For this review, use the dimensioned drawing (mm, ordinates from the lowest corner) and the shaded views. A direction names the side the tool comes from. Coordinates: 2 decimals unless noted, no trailing zeros. Order: outer loops, then holes, each group sorted by start corner. A loop starts at its lowest first (then second) coordinate and runs counter-clockwise, first axis right, second up. Notation, with made-up numbers: M 78.5,15.5 L 118.5,15.5 A29 ccw 118.5,54.5 Z; hole C 52,77 d3. An arc over 180 degrees is marked long. Answer in a Markdown table with one row per item.
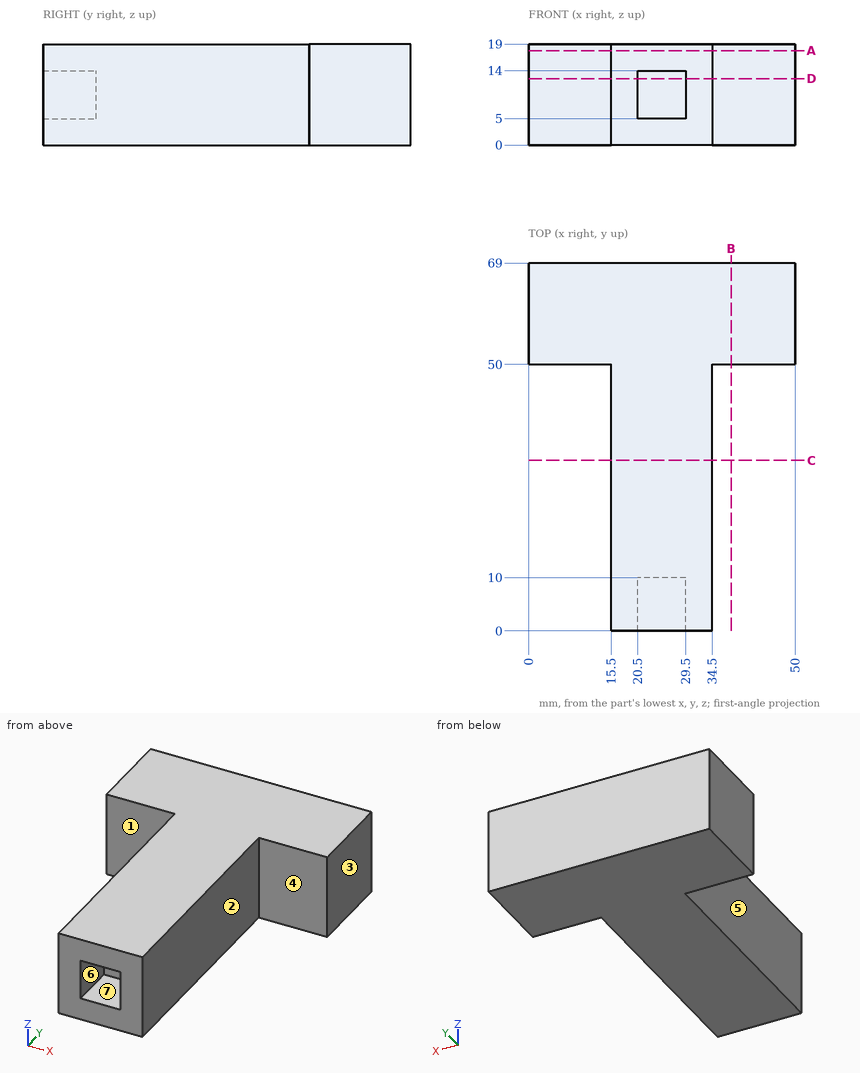
(1) Take a section at A-A (z = 17.75). Write out the cut boundary in (x, y).
Report:
| item | result |
|---|---|
| outline | M 0,50 L 15.5,50 L 15.5,0 L 34.5,0 L 34.5,50 L 50,50 L 50,69 L 0,69 Z |
(2) Machinability: for the marked faces 1, 2 and 3, which of the approach directions +Z, -Z, +X, -X, +Y, -Y give a long, thin tool a straight path to every point of the face, cutting with its end or side? Answer none if there is none.
Report:
| item | result |
|---|---|
| face 1 | +Z, -Z, -X, -Y |
| face 2 | +Z, -Z, +X, -Y |
| face 3 | +Z, -Z, +X, +Y, -Y |
(3) Take a section at C-C (y = 32). Write out the cut boundary in (x, z), then the cut area to 3 significant figures.
Report:
| item | result |
|---|---|
| outline | M 15.5,0 L 34.5,0 L 34.5,19 L 15.5,19 Z |
| area | 361 mm^2 |
(4) The part is to be moulded in two halves that separate along X. For the marked faces 4, 5, 6 and 7, say which applies: +X half, -X half, draft (parallel to the pull), parting line (faces both ways), or undercut.
Report:
| item | result |
|---|---|
| face 4 | draft |
| face 5 | -X half |
| face 6 | undercut |
| face 7 | undercut |
(5) To check wall thickness, follow line 1 (Y direction, x = 11.5, z = 7.5); line 2 (X direction, y = 24.5, z = 14.5); line 3 (Y direction, x = 24, z = 8). State the ranges of each line that lie inside material, in increasing order. Write a range as [from, to].
Report:
| item | result |
|---|---|
| line 1 | [50, 69] |
| line 2 | [15.5, 34.5] |
| line 3 | [10, 69] |
(6) Insertion check: P1, Ø6, axis at y = 40, z = 9, coming from the -X side; P2, Ø2.5, axis at x = 23.5, z = 9.5, coming from the -Y side; P3, Ø8, axis at x = 42, z = 10, coming from the -Y side; P4, Ø10, axis at x = 23, y = 7.5, coming from the -Z side. Each pin has a flat end and moves straight along its axis. Give the tip position at first contact, or say it passes through.
Report:
| item | result |
|---|---|
| P1 | x = 15.5 |
| P2 | y = 10 |
| P3 | y = 50 |
| P4 | z = 0 |
(7) Take a section at B-B (x = 38). Write out the cut boundary in (y, z), then the cut area to 3 significant figures.
Report:
| item | result |
|---|---|
| outline | M 50,0 L 69,0 L 69,19 L 50,19 Z |
| area | 361 mm^2 |
(8) Take a section at D-D (z = 12.5). Write out the cut boundary in (x, y).
Report:
| item | result |
|---|---|
| outline | M 0,50 L 15.5,50 L 15.5,0 L 20.5,0 L 20.5,10 L 29.5,10 L 29.5,0 L 34.5,0 L 34.5,50 L 50,50 L 50,69 L 0,69 Z |
